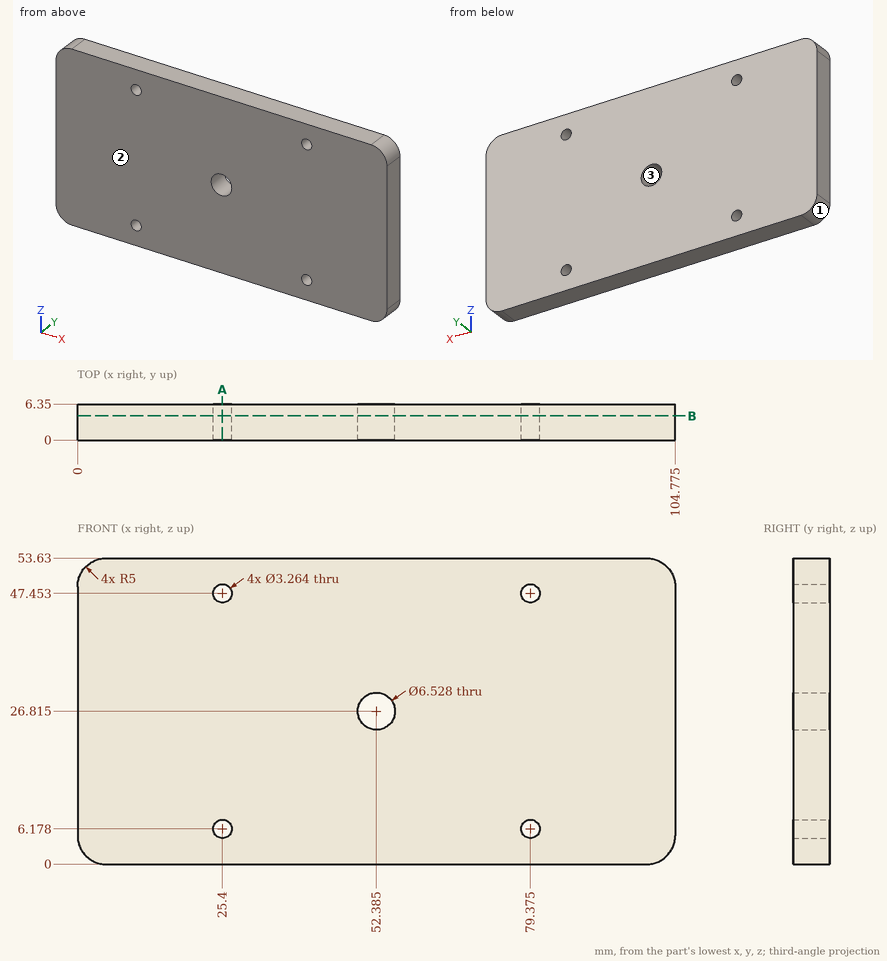
Geometry: see drawing. Coordinates: mm, zero at the bounding-box minimum. Coordinates: 2 decimals unless noted, no trailing zeros. Write each loop counter-clockwise with the first axis right and the second up, starting at its lowest first coordinate (ties: lowest second). Pieces come first, ordered by that corner, then holes.
1) Material intervals for line 1 along Z through (x, y) = (25.4, 2) (1 decimal); line 2 along X through (y, z) = (4.25, 26.5) (1 decimal); line 3 along Z through (x, y) = (49.5, 5) (1 decimal), sorted ascending.
2) Mould query, pull axis Z, two halves, no side actions, for the marked faces 1, 2 and 3. Classes: pulls with the +Z half, pulls with the -Z half, needs draft (parallel to the pull), parting line crosses it, or undercut.
3) Section B-B on y = 4.25. Output: boundary loops of the cut face in (x, z) (1 decimal).
4) Section A-A on x = 25.4. State how many separate pieces and enclosed holes the cut face has, and give its area (3 significant figures).
Check result:
1. line 1: z = 0 to 4.5, 7.8 to 45.8, 49.1 to 53.6
1. line 2: x = 0 to 49.1, 55.6 to 104.8
1. line 3: z = 0 to 25.3, 28.3 to 53.6
2. face 1: pulls with the -Z half
2. face 2: needs draft
2. face 3: undercut
3. outline: (0, 5) arc R5 ccw to (5, 0) - (99.8, 0) arc R5 ccw to (104.8, 5) - (104.8, 48.6) arc R5 ccw to (99.8, 53.6) - (5, 53.6) arc R5 ccw to (0, 48.6) - close; hole circle Ø3.3 at (25.4, 6.2); hole circle Ø3.3 at (25.4, 47.5); hole circle Ø6.5 at (52.4, 26.8); hole circle Ø3.3 at (79.4, 6.2); hole circle Ø3.3 at (79.4, 47.5)
4. separate pieces: 3
4. enclosed holes: 0
4. area: 299 mm2
